Autodesk Inventor part; units mm, degrees
ref_plane "YZ Plane" through (0, 0, 0) normal (1, 0, 0) x (0, 1, 0)
ref_plane "XZ Plane" through (0, 0, 0) normal (0, 1, 0) x (-1, 0, 0)
ref_plane "XY Plane" through (0, 0, 0) normal (0, 0, 1) x (1, 0, 0)
sketch "Sketch1" plane through (0, 0, 0) normal (0, 0, 1) x (1, 0, 0)
  circle A0 centre (0, 0) radius 3
  circle A1 centre (0, 0) radius 1.5
  dimension "d0" = 6
  dimension "d1" = 3
extrude "Extrusion1" add sketch "Sketch1" along normal blind 25 contours A0 | A1
extrude "Extrusion2" cut sketch "Sketch1" along normal blind 10 contours A1
extrude "Extrusion3" add sketch "Sketch1" along normal blind 8 from surface at 25 contours A1
thread "Thread1"
thread "Thread2"
properties part number "Abstandsbolzen PA6.6 schwarz IA Ø6x20 I=M3x10 A=M3x8 o. Freistich"
For this review, take the finished solid that the model builds, in its own axes (mm). A direction names the side the tool comes from. Round coordinates to 2 decimals unless told otherwise and drop trailing zeros. Loops run counter-clockwise (first coordinate to the right, second up) from the corner with the lowest first, then second, coordinate; pieces in that order, holes last.
Q1. Add section C-C on z = 12.5. Write out the cut boundary in (x, y).
Result sheet:
outline: circle Ø6 at (0, 0)
Q2. Machinability: for faces 1 (the face through (1.3, -1.3, 0)), 2 (the face through (0, 0, 10)), 3 (the face through (-1.5, -0.07, 28.94)), which of the approach directions +Z, -Z, +X, -X, +Y, -Y give a long, thin tool a straight path to every point of the face, cutting with its end or side? Answer none if there is none.
Result sheet:
face 1: -Z, +X, -X, +Y, -Y
face 2: -Z
face 3: +Z
Q3. Add section A-A on x = 0. Write out the cut boundary in (y, z), plus the area to 3 significant figures.
Result sheet:
outline: (-3, 0) - (-1.5, 0) - (-1.5, 10) - (1.5, 10) - (1.5, 0) - (3, 0) - (3, 25) - (1.5, 25) - (1.5, 33) - (-1.5, 33) - (-1.5, 25) - (-3, 25) - close
area: 144 mm2
Q4. Mouldability with a two-part tool opening along Y and no side actions: class faces 4 (the face through (-1.5, -0.07, 4.93)), 5 (the face through (0, 0, 33)), 6 (the face through (-3, 0, 12)) as +Y half, -Y half, draft (parallel to the pull), parting line (faces both ways), or undercut.
Result sheet:
face 4: undercut
face 5: draft
face 6: parting line
Q5. To check wall thickness, follow line 1 along Y through (x, z) = (0, 7); line 2 along Z through (x, y) = (1, -2.15); line 3 along Z through (x, y) = (-0.15, -0.2). State the ranges of each line that lie inside material, in increasing order.
Result sheet:
line 1: y = -3 to -1.5, 1.5 to 3
line 2: z = 0 to 25
line 3: z = 10 to 33
Q6. Insertion check: pin 1 Ø1 at (y, z) = (0.5, 26.5) entering from -X. The pin has a flat end and moves straight along its axis. Give the tip position at first contact, or say it passes through.
Result sheet:
pin 1: stops at x = -1.5
Q7. Add section D-D on x = -2.4. Write out the cut boundary in (y, z), plus the area to 3 significant figures.
Result sheet:
outline: (-1.8, 0) - (1.8, 0) - (1.8, 25) - (-1.8, 25) - close
area: 90.0 mm2
